Input: part model. Units: mm. Frame: model coordinates. Face numbers are marked on the shaded views. Round coordinates to 2 decimals unless told otherwise and drop trailing zeros. Order: outer loops, then holes, each group sorted by start corner. A loop starts at its lowest first (then second) coordinate and runs counter-clockwise, first axis right, second up. Notation, with made-up numbers: (14.5, -20) -> (19.5, -20) arc R38 ccw to (19.5, 19) -> close; hole circle Ø9 at (72, 43.25). An arc over 180 degrees is marked (long way). Use a Markdown table: item, result.
from build123d import *

# Parameters (mm, degrees)
SKETCH1_W                 = 44.04
SKETCH1_H                 = 10
BOSS_EXTRUDE1_DEPTH       = 4.7625
SKETCH2_R                 = 1.03
CUT_EXTRUDE1_DEPTH        = 25.648768859
F_1_64_TAPPED_HOLE1_D     = 1.5113
F_1_64_TAPPED_HOLE1_DEPTH = 6.35
F_1_64_TAPPED_HOLE1_TIP   = 0.454040327
F_1_64_TAPPED_HOLE2_D     = 1.5113
F_1_64_TAPPED_HOLE2_DEPTH = 6.35
F_1_64_TAPPED_HOLE2_TIP   = 0.454040327
SKETCH7_W                 = 22
SKETCH7_H                 = 3.65
CUT_EXTRUDE2_DEPTH        = 10
FILLET1_R                 = 4
FILLET2_R                 = 4


with BuildPart() as part:
    # Sketch1 → Boss-Extrude1 (new body)
    with BuildSketch(Plane.XY):
        Rectangle(SKETCH1_W, SKETCH1_H)
    extrude(amount=BOSS_EXTRUDE1_DEPTH)

    # Sketch2 → Cut-Extrude1 (cut, through all)
    with BuildSketch(Plane(origin=(0, 5, 0), x_dir=(1, 0, 0), z_dir=(0, 1, 0))):
        with Locations(Location((-5, -2.38125, 0), (0, 0, 270))):
            Circle(SKETCH2_R)
        with Locations(Location((5, -2.38125, 0), (0, 0, 270))):
            Circle(SKETCH2_R)
    extrude(amount=-CUT_EXTRUDE1_DEPTH, mode=Mode.SUBTRACT)

    # #1-64 Tapped Hole1
    with Locations(Plane.ZY.offset(22.02)):
        with Locations((2.38125, 3.5), (2.38125, 0)):
            Hole(F_1_64_TAPPED_HOLE1_D / 2, depth=F_1_64_TAPPED_HOLE1_DEPTH)
            with Locations((0, 0, -(F_1_64_TAPPED_HOLE1_DEPTH + F_1_64_TAPPED_HOLE1_TIP / 2))):  # 118° drill point
                Cone(0, F_1_64_TAPPED_HOLE1_D / 2, F_1_64_TAPPED_HOLE1_TIP, mode=Mode.SUBTRACT)

    # #1-64 Tapped Hole2
    with Locations(Plane(origin=(22.02, 0, 0), x_dir=(0, 0, -1), z_dir=(1, 0, 0))):
        with Locations((-2.38125, 3.5), (-2.38125, 0)):
            Hole(F_1_64_TAPPED_HOLE2_D / 2, depth=F_1_64_TAPPED_HOLE2_DEPTH)
            with Locations((0, 0, -(F_1_64_TAPPED_HOLE2_DEPTH + F_1_64_TAPPED_HOLE2_TIP / 2))):  # 118° drill point
                Cone(0, F_1_64_TAPPED_HOLE2_D / 2, F_1_64_TAPPED_HOLE2_TIP, mode=Mode.SUBTRACT)

    # Sketch7 → Cut-Extrude2 (cut)
    with BuildSketch(Plane.XY.offset(4.7625)):
        with Locations((0, 3.175)):
            Rectangle(SKETCH7_W, SKETCH7_H)
    extrude(amount=-CUT_EXTRUDE2_DEPTH, mode=Mode.SUBTRACT)

    # Fillet1
    # the kernel refuses this fillet: 4 mm, written as the material it takes off along each edge
    with BuildSketch(Plane(origin=(11, 5, 14.724145195), x_dir=(0, -1, 0), z_dir=(0, 0, -1))) as fillet1_piece_1:
        with BuildLine():
            CenterArc((4, -3.984658078), FILLET1_R, 95.019800132, 84.980199868)
            Line((0, -3.984658078), (-0.08, -3.984658078))
            Line((-0.08, -3.984658078), (-0.08, 0))
            Line((-0.08, 0), (0, 0.08))
            ThreePointArc((0, 0.08), (1.825, 0.08), (3.643, 0.079693162))
            Line((3.643, 0.079693162), (3.65, 0))
        make_face()
    extrude(amount=24.685790391, mode=Mode.SUBTRACT)
    with BuildSketch(Plane(origin=(-11, 5, 14.724145195), x_dir=(-1, 0, 0), z_dir=(0, 0, -1))) as fillet1_piece_2:
        with BuildLine():
            CenterArc((3.984658078, -4), FILLET1_R, 90, 84.980199868)
            Line((0, -3.65), (-0.079693162, -3.643))
            ThreePointArc((-0.079693162, -3.643), (-0.08, -1.825), (-0.08, 0))
            Line((-0.08, 0), (0, 0.08))
            Line((0, 0.08), (3.984658078, 0.08))
            Line((3.984658078, 0.08), (3.984658078, 0))
        make_face()
    extrude(amount=24.685790391, mode=Mode.SUBTRACT)

    # Fillet2
    fillet2_edges = [part.edges().sort_by_distance(p)[0] for p in [
        (11, 1.35, 2.38125),
        (-11, 1.35, 2.38125),
    ]]
    fillet(fillet2_edges, radius=FILLET2_R)


solid = part.part
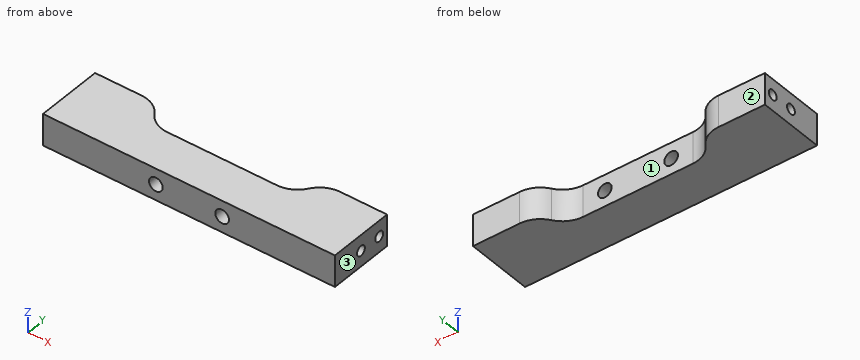
1) Pin query (flat end, axial travel): pin 1 Ø1.9 at (x, z) = (5, 2.38) entering from +Y; pin 2 Ø1.5 at (x, z) = (4.5, 3) entering from +Y; pin 3 Ø1.4 at (y, z) = (3.5, 2.38) entering from +X. Return the tip coordinate at first contact, or that it passes through.
Results found:
| item | result |
|---|---|
| pin 1 | passes through |
| pin 2 | stops at y = 1.35 |
| pin 3 | stops at x = 15.64 |
2) Pull-direction query (X, two-part tool) for the marked faces 1, 2 and 3; classes: +X half, -X half, draft (parallel to the pull), parting line (faces both ways), or undercut.
Results found:
| item | result |
|---|---|
| face 1 | undercut |
| face 2 | draft |
| face 3 | +X half |
3) Cut plane A-A on x = 5. Return loops of the section in (y, z).
Results found:
| item | result |
|---|---|
| outline | (-5, 0) -> (1.35, 0) -> (1.35, 1.35) -> (-5, 1.35) -> close; (-5, 3.41) -> (1.35, 3.41) -> (1.35, 4.76) -> (-5, 4.76) -> close |
4) Line query: L1, parallel to Y at x = -18.5, z = 2.4; L2, parallel to X at y = -3.5, z = 2.4; L3, parallel to Y at x = -17.5, z = 1.8. Output: solid intervals per line, ascending. Write a range as [from, to].
Results found:
| item | result |
|---|---|
| L1 | y = [-5, -0.76], [0.76, 2.74], [4.26, 5] |
| L2 | x = [-22.02, -6.03], [-3.97, 3.97], [6.03, 22.02] |
| L3 | y = [-5, -0.48], [0.48, 3.02], [3.98, 5] |
5) Cut plane C-C on z = 0.75. Return loops of the section in (x, y) (3 decimals), and give its area (3 significant figures).
Results found:
| item | result |
|---|---|
| outline | (-22.02, -5) -> (22.02, -5) -> (22.02, 5) -> (14.985, 5) arc R4 ccw to (11.628, 3.175) arc R4 cw to (8.271, 1.35) -> (-8.271, 1.35) arc R4 cw to (-11.628, 3.175) arc R4 ccw to (-14.985, 5) -> (-22.02, 5) -> close |
| area | 356 mm² |
6) Cut plane B-B on y = -3.5. Return loops of the section in (x, z), and give its area (3 significant figures).
Results found:
| item | result |
|---|---|
| outline | (-22.02, 0) -> (22.02, 0) -> (22.02, 4.76) -> (-22.02, 4.76) -> close; hole circle Ø2.06 at (-5, 2.38); hole circle Ø2.06 at (5, 2.38) |
| area | 203 mm² |
